Verification items for the finished model (mm, model axes). Give positions to 0.01 mm unless a question says otherwise; leave off trailing zeros. Write each loop counter-clockwise with the first axis right and the second up, starting at its lowest first coordinate (ties: lowest second). Pieces come first, ordered by that corner, then holes. Notation, with made-up numbers: M -15.75,-27.5 L 0.25,-27.5 A27 ccw 0.25,-9.5 Z; hole C -29.75,73 d4. An arc over 180 degrees is marked long. Answer as a JSON object with one key per item and string values.
```python
from build123d import *

# Parameters (mm, degrees)
F0_R     = 4.9657
F1_DEPTH = 6.35
F2_R     = 5.08


# Not quite as in the source:
# - a feature names something its author has since deleted; it is built from what else it names


with BuildPart() as f1:
    # F0 (on Front) → F1 (new body)
    with BuildSketch(Plane.XZ):
        Polygon((-120.1667662859, -0.1937935591), (16.3582337141, -0.1937935591), (16.3582337141, 82.3562064409), (-37.6167662859, 163.3187064409), (-120.1667662859, 163.3187064409), (-120.1667662859, 144.2687064409), align=None)
        with Locations((-93.1792662859, 42.6687064409)):
            Circle(F0_R, mode=Mode.SUBTRACT)
        with Locations((-50.3167662859, 42.6687064409)):
            Circle(F0_R, mode=Mode.SUBTRACT)
        with Locations((-2.6917662859, 26.7937064409)):
            Circle(F0_R, mode=Mode.SUBTRACT)
        with Locations((-2.6917662859, 69.6562064409)):
            Circle(F0_R, mode=Mode.SUBTRACT)
        with BuildLine():
            ThreePointArc((-88.2135662859, 144.2687064409), (-93.1792662859, 139.3030064409), (-98.1449662859, 144.2687064409))
            ThreePointArc((-98.1449662859, 144.2687064409), (-93.1792662859, 149.2344064409), (-88.2135662859, 144.2687064409))
        make_face(mode=Mode.SUBTRACT)
        with Locations((-50.3167662859, 144.2687064409)):
            Circle(F0_R, mode=Mode.SUBTRACT)
    extrude(amount=F1_DEPTH)

    # F2
    f2_edges = [f1.edges().sort_by_distance(p)[0] for p in [
        (-37.616766, -3.175, 163.318706),
        (16.358234, -3.175, 82.356206),
        (16.358234, -3.175, -0.193794),
        (-120.166766, -3.175, -0.193794),
        (-120.166766, -3.175, 163.318706),
    ]]
    fillet(f2_edges, radius=F2_R)


solid = f1.part
```
1) Section check C-C on z = 130. Record the boundary of the cut face in (x, y), and give its area (3 significant figures).
Completed:
{"outline": "M -120.17,-6.35 L -15.4,-6.35 L -15.4,0 L -120.17,0 Z", "area": "665 mm2"}
2) Release check for a two-part mould opening along X. For faces 1 (the face through (-90.89, -3.13, 38.26)), 2 (the face through (-53, -3, -0.194)), 3 (the face through (16.358, -3, 42)) record: pulls with the +X half, pulls with the -X half, needs draft (parallel to the pull), parting line crosses it, or undercut.
Completed:
{"face 1": "undercut", "face 2": "needs draft", "face 3": "pulls with the +X half"}
3) Section check A-A on x = -91. Record the boundary of the cut face in (y, z), and give its area (3 significant figures).
Completed:
{"outline": "M -6.35,-0.19 L 0,-0.19 L 0,38.21 L -6.35,38.21 Z; M -6.35,47.13 L 0,47.13 L 0,139.81 L -6.35,139.81 Z; M -6.35,148.73 L 0,148.73 L 0,163.32 L -6.35,163.32 Z", "area": "925 mm2"}
4) Go/stop test with a flat-tipped pin: pin 1 (2 mm diameter, centred on x = -83, z = 69, fed in from +Y). Record where the tip stops, or that it passes through.
Completed:
{"pin 1": "stops at y = 0"}
5) Section check B-B on y = -5. Record the boundary of the cut face in (x, z), and give its area (3 significant figures).
Completed:
{"outline": "M -120.17,4.89 A5.08 ccw -115.09,-0.19 L 11.28,-0.19 A5.08 ccw 16.36,4.89 L 16.36,80.82 A5.08 ccw 15.51,83.64 L -36.11,161.06 A5.08 ccw -40.34,163.32 L -115.09,163.32 A5.08 ccw -120.17,158.24 Z; hole C -93.18,42.67 d9.93; hole C -93.18,144.27 d9.93; hole C -50.32,42.67 d9.93; hole C -50.32,144.27 d9.93; hole C -2.69,26.79 d9.93; hole C -2.69,69.66 d9.93", "area": "19,700 mm2"}
6) Section check D-D on x = -11. Record the boundary of the cut face in (y, z), and give its area (3 significant figures).
Completed:
{"outline": "M -6.35,-0.19 L 0,-0.19 L 0,123.39 L -6.35,123.39 Z", "area": "785 mm2"}
7) Thickness scan on L1, parallel to X at y = -4.75, z = 142; L2, parallel to X at y = -1, z = 26.5; L3, parallel to Z at x = -0.5, y = -0.75. Record the ranges inside material, lowest first.
Completed:
{"L1": "x = -120.17 to -97.6, -88.76 to -54.73, -45.9 to -23.4", "L2": "x = -120.17 to -7.65, 2.27 to 16.36", "L3": "z = -0.19 to 22.34, 31.25 to 65.2, 74.11 to 107.64"}
